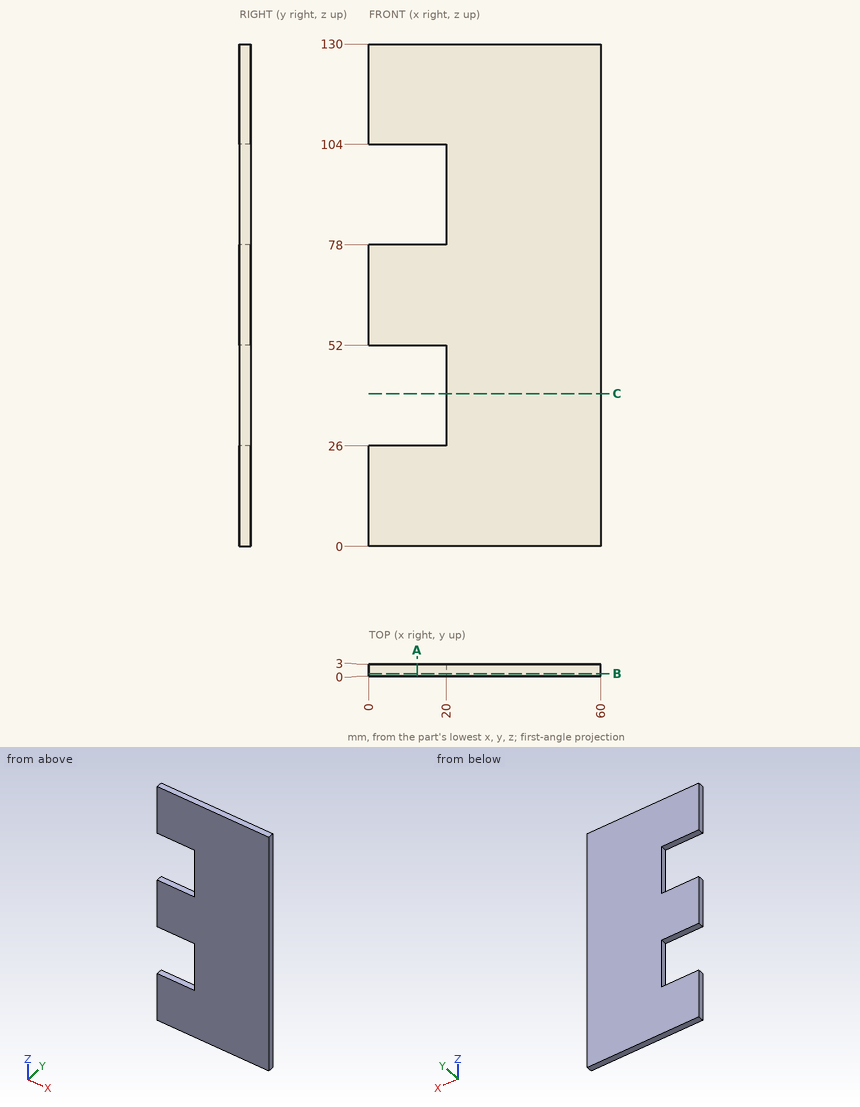
Verification items for this drawing (mm, ordinates from the low corner). Give positions to 0.01 mm unless a question says otherwise; leave off trailing zeros. Write each loop counter-clockwise with the first axis right and the second up, starting at its lowest first coordinate (ties: lowest second). Pieces come first, ordered by that corner, then holes.
1) Section check B-B, the plane y = 0.6. Record the boundary of the cut face in (x, z).
2) Material ranges on L1, parallel to Z at x = 6, y = 0.8; L2, parallel to X at y = 1.2, z = 81, recorded low to high.
3) Section check C-C, the plane z = 39.5. Record the boundary of the cut face in (x, y).
4) Gauge pin test, flat ends, axial feed: pin 1 (0.9 mm diameter, centred on y = 1, z = 95, fed in from -X); pin 2 (6 mm diameter, centred on x = 40, z = 49, fed in from -Y); pin 3 (3 mm diameter, centred on x = 11.5, z = 101.5, fed in from -Y). Record the tip position at first contact, or that the pin passes through.
5) Section check A-A, the plane x = 12.5. Record the boundary of the cut face in (y, z).
Computed:
1. outline: (0, 0) - (60, 0) - (60, 130) - (0, 130) - (0, 104) - (20, 104) - (20, 78) - (0, 78) - (0, 52) - (20, 52) - (20, 26) - (0, 26) - close
2. L1: z = 0 to 26, 52 to 78, 104 to 130
2. L2: x = 20 to 60
3. outline: (20, 0) - (60, 0) - (60, 3) - (20, 3) - close
4. pin 1: stops at x = 20
4. pin 2: stops at y = 0
4. pin 3: passes through
5. outline: (0, 0) - (3, 0) - (3, 26) - (0, 26) - close; (0, 52) - (3, 52) - (3, 78) - (0, 78) - close; (0, 104) - (3, 104) - (3, 130) - (0, 130) - close
